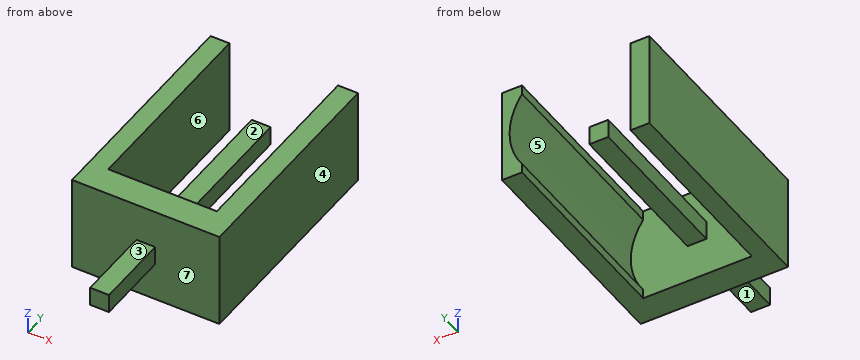
from build123d import *

# Parameters (mm, degrees)
SKETCH_1_W             = 7.8
SKETCH_1_H             = 5.08
EXTRUDE_1_DEPTH        = 12
CUT_EXTRUDE_1_DEPTH    = 10.5
EXTRUDE_1_2_DEPTH      = 4
EXTRUDE_1_2_DEPTH_BACK = 10
SKETCH_4_W             = 1
SKETCH_4_H             = 1


with BuildPart() as part:
    # 草图1 → Extrude 1 (new body)
    with BuildSketch(Plane(origin=(0, 0, 0), x_dir=(1, 0, 0), z_dir=(0, 1, 0))):
        Rectangle(SKETCH_1_W, SKETCH_1_H)
    extrude(amount=EXTRUDE_1_DEPTH)

    # 草图2 → 切除-拉伸1 (cut)
    with BuildSketch(Plane(origin=(0, 12, 0), x_dir=(-1, 0, 0), z_dir=(0, 1, 0))):
        with BuildLine():
            Line((-2.844011252, 2.04), (-2.844011252, 2.54))
            Line((-2.844011252, 2.54), (2.9, 2.54))
            Line((2.9, 2.54), (2.9, -2.54))
            Line((2.9, -2.54), (-2.844011252, -2.54))
            Line((-2.844011252, -2.54), (-2.844011252, -2.04))
            ThreePointArc((-2.844011252, -2.04), (-3.5, 0), (-2.844011252, 2.04))
        make_face()
    extrude(amount=-CUT_EXTRUDE_1_DEPTH, mode=Mode.SUBTRACT)

    # 草图4 → Extrude 1 2 (add, two sides: drawn at the far end of the back side and taken through both)
    with BuildSketch(Plane.XZ.offset(-EXTRUDE_1_2_DEPTH_BACK)):
        Rectangle(SKETCH_4_W, SKETCH_4_H)
    extrude(amount=EXTRUDE_1_2_DEPTH + EXTRUDE_1_2_DEPTH_BACK)


solid = part.part
Input: part model. Units: mm. Frame: model coordinates. Face numbers are marked on the shaded views. A direction names the side the tool comes from. Give positions to 0.01 mm unless a question says otherwise; leave off trailing zeros. Write each loop counter-clockwise with the first axis right and the second up, starting at its lowest first coordinate (ties: lowest second). Pieces come first, ordered by that corner, then holes.
Q1. Section C-C, the plane x = -0.25. Output: boundary loops of the cut face in (y, z).
Q2. First-contact query: P1, Ø1, axis at x = -1.5, z = -0.5, coming from the +Y side; P2, Ø1.1, axis at x = 0, y = -1.5, coming from the +Z side; P3, Ø0.5, axis at x = 0, y = 5.5, coming from the -Z side. Flat tips, straight axial feed; report the tip coordinate or a pass-through.
Q3. Section B-B, the plane y = 3.5. Output: boundary loops of the cut face in (x, z), plus the area to 3 significant figures.
Q4. Section D-D, the plane z = -0.3. Output: boundary loops of the cut face in (x, y).
Q5. Section A-A, the plane y = 10.5. Output: boundary loops of the cut face in (x, z).
Q6. Material intervals for probe 1 along Y at (x, z) = (-1.75, 1.9); probe 2 along Y at (x, z) = (-3.25, 0.7); probe 3 along X at (y, z) = (4, -0.2), sorted ascending.
Q7. Pull-direction query (X, two-part tool) for the marked faces 4, 5, 6 and 7; classes: pulls with the +X half, pulls with the -X half, needs draft (parallel to the pull), parting line crosses it, or undercut.
Q8. Set-up query: the marked faces 1, 2 and 3. Return all of +Z, -Z, +X, -X, +Y, -Y with unobstructed straight access to the full face (end or side cutting, diameter ignored); none if empty.
Filled in:
1. outline: (-4, -0.5) - (0, -0.5) - (0, -2.54) - (1.5, -2.54) - (1.5, -0.5) - (10, -0.5) - (10, 0.5) - (1.5, 0.5) - (1.5, 2.54) - (0, 2.54) - (0, 0.5) - (-4, 0.5) - close
2. P1: stops at y = 1.5
2. P2: stops at z = 0.5
2. P3: stops at z = -0.5
3. outline: (-3.9, -2.54) - (-2.9, -2.54) - (-2.9, 2.54) - (-3.9, 2.54) - close; (-0.5, -0.5) - (0.5, -0.5) - (0.5, 0.5) - (-0.5, 0.5) - close; (2.84, -2.54) - (3.9, -2.54) - (3.9, 2.54) - (2.84, 2.54) - (2.84, 2.04) arc R3.5 cw to (2.84, -2.04) - close
3. area: 9.62 mm2
4. outline: (-3.9, 0) - (-0.5, 0) - (-0.5, -4) - (0.5, -4) - (0.5, 0) - (3.9, 0) - (3.9, 12) - (3.49, 12) - (3.49, 1.5) - (0.5, 1.5) - (0.5, 10) - (-0.5, 10) - (-0.5, 1.5) - (-2.9, 1.5) - (-2.9, 12) - (-3.9, 12) - close
5. outline: (-3.9, -2.54) - (-2.9, -2.54) - (-2.9, 2.54) - (-3.9, 2.54) - close; (2.84, -2.54) - (3.9, -2.54) - (3.9, 2.54) - (2.84, 2.54) - (2.84, 2.04) arc R3.5 cw to (2.84, -2.04) - close
6. probe 1: y = 0 to 1.5
6. probe 2: y = 0 to 12
6. probe 3: x = -3.9 to -2.9, -0.5 to 0.5, 3.49 to 3.9
7. face 4: pulls with the +X half
7. face 5: undercut
7. face 6: undercut
7. face 7: needs draft
8. face 1: -Z, +X, -X, -Y
8. face 2: +Z, +Y
8. face 3: +Z, +X, -X, -Y
